from build123d import *

# Parameters (mm, degrees)
F0_W      = 40
F0_H      = 40
F1_DEPTH  = 10
F3_D      = 5
F4_R      = 9
F4_R_2    = 7.75
F5_DEPTH  = 5
F7_D      = 5.1054
F7_DEPTH  = 5
F7_TIP    = 1.5338169022
F9_D      = 5.1054
F9_DEPTH  = 5
F9_TIP    = 1.5338169022
F11_D     = 5.1054
F11_DEPTH = 5
F11_TIP   = 1.5338169022
F13_D     = 5.1054
F13_DEPTH = 5
F13_TIP   = 1.5338169022


with BuildPart() as f1:
    # F0 (on Front) → F1 (new body)
    with BuildSketch(Plane.XZ):
        Rectangle(F0_W, F0_H)
    extrude(amount=F1_DEPTH)

    # F3 (through all)
    with Locations(Plane.XZ.offset(10)):
        with Locations((0, 0)):
            Hole(F3_D / 2)

    # F4 (on face) → F5 (cut)
    with BuildSketch(Plane.XZ.offset(10)):
        Circle(F4_R)
        Circle(F4_R_2, mode=Mode.SUBTRACT)
    extrude(amount=-F5_DEPTH, mode=Mode.SUBTRACT)

    # F7
    with Locations(Plane.XY.offset(20)):
        with Locations((0, -5)):
            Hole(F7_D / 2, depth=F7_DEPTH)
            with Locations((0, 0, -(F7_DEPTH + F7_TIP / 2))):  # 118° drill point
                Cone(0, F7_D / 2, F7_TIP, mode=Mode.SUBTRACT)

    # F9
    with Locations(Plane(origin=(0, 0, -20), x_dir=(1, 0, 0), z_dir=(0, 0, -1))):
        with Locations((0, 5)):
            Hole(F9_D / 2, depth=F9_DEPTH)
            with Locations((0, 0, -(F9_DEPTH + F9_TIP / 2))):  # 118° drill point
                Cone(0, F9_D / 2, F9_TIP, mode=Mode.SUBTRACT)

    # F11
    with Locations(Plane(origin=(-20, 0, 0), x_dir=(0, -1, 0), z_dir=(-1, 0, 0))):
        with Locations((5, 0)):
            Hole(F11_D / 2, depth=F11_DEPTH)
            with Locations((0, 0, -(F11_DEPTH + F11_TIP / 2))):  # 118° drill point
                Cone(0, F11_D / 2, F11_TIP, mode=Mode.SUBTRACT)

    # F13
    with Locations(Plane.YZ.offset(20)):
        with Locations((-5, 0)):
            Hole(F13_D / 2, depth=F13_DEPTH)
            with Locations((0, 0, -(F13_DEPTH + F13_TIP / 2))):  # 118° drill point
                Cone(0, F13_D / 2, F13_TIP, mode=Mode.SUBTRACT)


solid = f1.part
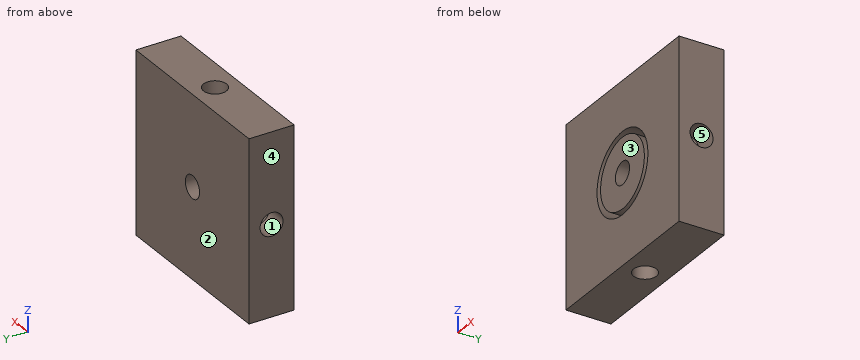
Model file for the job. Use its own axes, mm. Face numbers are marked on the shaded views. A direction names the side the tool comes from. Give positions to 0.01 mm unless a question says otherwise; leave off trailing zeros. Write each loop counter-clockwise with the first axis right and the second up, starting at its lowest first coordinate (ties: lowest second). Pieces come first, ordered by that corner, then holes. Notation, with made-up numbers: (12.25, -13) -> (28.25, -13) arc R23 cw to (28.25, 9) -> close; hole circle Ø1 at (66, 42). An arc over 180 degrees is marked (long way). Write item = value, one per line.
(1) Tool access for the marked faces 1 and 2: list every direction of +Z, -Z, +X, -X, +Y, -Y with a clear straight run to the whole face (end or side of a thin tool).
Determined:
face_1 = -X
face_2 = +Z, -Z, +X, -X, +Y
(2) Probe line 1 along Z through (x, y) = (0, -8.25); line 2 along Z through (x, y) = (0, -5.5); line 3 along Z through (x, y) = (-16.45, -5). List the from-to ranges inside material, lowest first.
Determined:
line_1 = -20 to -9, -7.75 to -2.5, 2.5 to 7.75, 9 to 20
line_2 = -13.77 to -9, -7.75 to -2.5, 2.5 to 7.75, 9 to 13.77
line_3 = -20 to -2.55, 2.55 to 20
(3) Flat gauge pin, fed straight in: P1, Ø4.5, axis at x = 0, y = -5, coming from the +Z side. Where does the tip first touch, or does it go through?
Determined:
P1 = 14.82
(4) Slice it at B-B, the plane x = 16. Give the cut face in (y, z), then the cut area to 3 significant figures.
Determined:
outline = (-10, -20) -> (0, -20) -> (0, 20) -> (-10, 20) -> close; hole circle Ø5.11 at (-5, 0)
area = 380 mm2
(5) Slice it at C-C, the plane y = -6.5. Give the number of separate pieces and of enclosed holes in the cut face, then the cut area to 3 significant figures.
Determined:
separate_pieces = 2
enclosed_holes = 2
area = 1,430 mm2
(6) Mould opens along Y. For the marked faces 3, 4 and 5 say: released by +Y, released by -Y, zero draft, split by the parting line, or undercut.
Determined:
face_3 = released by -Y
face_4 = zero draft
face_5 = undercut
(7) Slice it at D-D, the plane z = -8.5. Give the cut face in (x, y).
Determined:
outline = (-20, -10) -> (-2.96, -10) -> (-2.96, -5) -> (2.96, -5) -> (2.96, -10) -> (20, -10) -> (20, 0) -> (-20, 0) -> close
(8) Slice it at A-A, the plane z = 16. Give the cut face in (x, y), then the cut area to 3 significant figures.
Determined:
outline = (-20, -10) -> (20, -10) -> (20, 0) -> (-20, 0) -> close; hole circle Ø5.11 at (0, -5)
area = 380 mm2
